Can you work these out from the model? Positions are in its coordinate system, mm. Face numbers are marked on the shaded views. A direction names the side the tool comes from. Coordinates: 2 decimals unless noted, no trailing zeros. Order: outer loops, then holes, each group sorted by start corner. A loop starts at its lowest first (then second) coordinate and runs counter-clockwise, first axis right, second up. Notation, with made-up numbers: M -6.75,28.5 L 45.25,28.5 A22 ccw 45.25,50.5 Z; hole C 8.25,9 d7. An arc over 180 degrees is marked long. Answer as a JSON object with one key per item and string values.
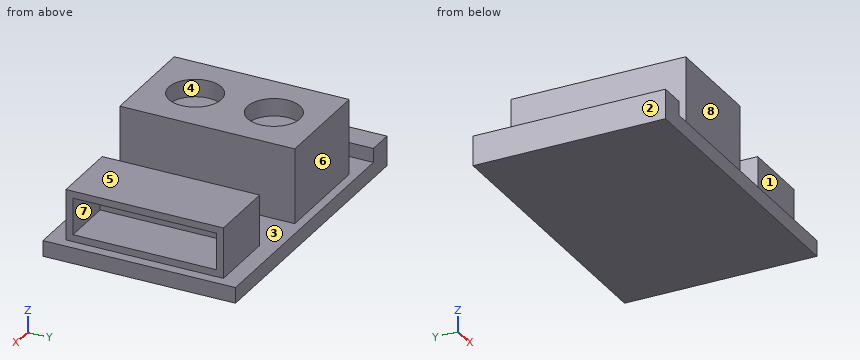
from build123d import *

# Parameters (mm, degrees)
ESBO_O1_W                = 16.7
ESBO_O1_H                = 11
RESSALTO_EXTRUS_O1_DEPTH = 5.2
ESBO_O2_W                = 16.7
ESBO_O2_H                = 11
ESBO_O2_W_2              = 6
ESBO_O2_H_2              = 10
ESBO_O2_W_3              = 4
ESBO_O2_H_3              = 9
CORTE_EXTRUS_O1_DEPTH    = 4.3
ESBO_O3_W                = 4
ESBO_O3_H                = 9
CORTE_EXTRUS_O2_DEPTH    = 1.4
ESBO_O4_R                = 1.5
CORTE_EXTRUS_O3_DEPTH    = 1
ESBO_O5_W                = 2.1
ESBO_O5_H                = 8.2
CORTE_EXTRUS_O4_DEPTH    = 3
ESBO_O6_W                = 1.5
ESBO_O6_H                = 11
RESSALTO_EXTRUS_O2_DEPTH = 0.8


with BuildPart() as part:
    # Esboço1 → Ressalto-extrusão1 (new body)
    with BuildSketch(Plane.XY):
        with Locations((3.068373494, 1.240361446)):
            Rectangle(ESBO_O1_W, ESBO_O1_H)
    extrude(amount=RESSALTO_EXTRUS_O1_DEPTH)

    # Esboço2 → Corte-extrusão1 (cut)
    with BuildSketch(Plane.XY.offset(5.2)):
        with Locations((3.068373494, 1.240361446)):
            Rectangle(ESBO_O2_W, ESBO_O2_H)
        with Locations((0.918373494, 1.240361446)):
            Rectangle(ESBO_O2_W_2, ESBO_O2_H_2, mode=Mode.SUBTRACT)
        with Locations((8.818373494, 1.240361446)):
            Rectangle(ESBO_O2_W_3, ESBO_O2_H_3, mode=Mode.SUBTRACT)
    extrude(amount=-CORTE_EXTRUS_O1_DEPTH, mode=Mode.SUBTRACT)

    # Esboço3 → Corte-extrusão2 (cut)
    with BuildSketch(Plane.XY.offset(5.2)):
        with Locations((8.818373494, 1.240361446)):
            Rectangle(ESBO_O3_W, ESBO_O3_H)
    extrude(amount=-CORTE_EXTRUS_O2_DEPTH, mode=Mode.SUBTRACT)

    # Esboço4 → Corte-extrusão3 (cut)
    with BuildSketch(Plane.XY.offset(5.2)):
        with Locations((0.918373494, 3.490361446)):
            Circle(ESBO_O4_R)
        with Locations((0.918373494, -1.009638554)):
            Circle(ESBO_O4_R)
    extrude(amount=-CORTE_EXTRUS_O3_DEPTH, mode=Mode.SUBTRACT)

    # Esboço5 → Corte-extrusão4 (cut)
    with BuildSketch(Plane(origin=(10.818373494, 0, 0), x_dir=(0, 0, -1), z_dir=(1, 0, 0))):
        with Locations((-2.35, 1.240361446)):
            Rectangle(ESBO_O5_W, ESBO_O5_H)
    extrude(amount=-CORTE_EXTRUS_O4_DEPTH, mode=Mode.SUBTRACT)

    # Esboço6 → Ressalto-extrusão2 (add)
    with BuildSketch(Plane.XY.offset(0.9)):
        with Locations((-4.531626506, 1.240361446)):
            Rectangle(ESBO_O6_W, ESBO_O6_H)
    extrude(amount=RESSALTO_EXTRUS_O2_DEPTH)


solid = part.part
Item 1: I want a section at B-B, the plane z = 2. Write out the boundary of the cut face in (x, y), plus the area to 3 significant figures.
Answers follow:
{"outline": "M -2.08,-3.76 L 3.92,-3.76 L 3.92,6.24 L -2.08,6.24 Z; M 6.82,-3.26 L 10.82,-3.26 L 10.82,-2.86 L 7.82,-2.86 L 7.82,5.34 L 10.82,5.34 L 10.82,5.74 L 6.82,5.74 Z", "area": "71.4 mm^2"}
Item 2: I want a section at A-A, the plane x = 8.75. Write out the boundary of the cut face in (y, z).
Answers follow:
{"outline": "M -4.26,0 L 6.74,0 L 6.74,0.9 L 5.74,0.9 L 5.74,3.8 L -3.26,3.8 L -3.26,0.9 L -4.26,0.9 Z; hole M -2.86,1.3 L 5.34,1.3 L 5.34,3.4 L -2.86,3.4 Z"}
Item 3: Please list where these lines run through material, in increasing order: line 1 (Z direction, x = 10.25, y = -2); line 2 (X direction, y = 0.75, z = 3.5); line 3 (X direction, y = -2.5, z = 2.45).
Answers follow:
{"line 1": "z = 0 to 1.3, 3.4 to 3.8", "line 2": "x = -2.08 to 3.92, 6.82 to 10.82", "line 3": "x = -2.08 to 3.92, 6.82 to 7.82"}
Item 4: If we mould it in two halves opening along X, with no side actions, what happens to the marked faces 1, 2 and 3? For each: pulls with the +X half, pulls with the -X half, needs draft (parallel to the pull), parting line crosses it, or undercut.
Answers follow:
{"face 1": "needs draft", "face 2": "pulls with the -X half", "face 3": "undercut"}
Item 5: Which directions (+Z, -Z, +X, -X, +Y, -Y) give clear straight access to the entire face, cutting with the end or side of a thin tool? Please do the marked faces 4, 5, 6, 7 and 8.
Answers follow:
{"face 4": "+Z", "face 5": "+Z, +X, +Y, -Y", "face 6": "+Z, +X, +Y", "face 7": "+X", "face 8": "+Z, +X, -Y"}
Item 6: I want a section at C-C, the plane y = 6. Write out the boundary of the cut face in (x, z), plus the area to 3 significant figures.
Answers follow:
{"outline": "M -5.28,0 L 11.42,0 L 11.42,0.9 L 3.92,0.9 L 3.92,5.2 L -2.08,5.2 L -2.08,0.9 L -3.78,0.9 L -3.78,1.7 L -5.28,1.7 Z", "area": "42.0 mm^2"}
Item 7: I want a section at D-D, the plane z = 4.55. Write out the boundary of the cut face in (x, y).
Answers follow:
{"outline": "M -2.08,-3.76 L 3.92,-3.76 L 3.92,6.24 L -2.08,6.24 Z; hole C 0.92,-1.01 d3; hole C 0.92,3.49 d3"}
Item 8: I'm going to push flat-ended pins straight in: pin 1 (2 mm diameter, centred on x = 1.5, z = 3, fed in from +Y); pin 2 (2.5 mm diameter, centred on y = -0.5, z = 2.5, fed in from -X); pin 3 (2 mm diameter, centred on y = 0.5, z = 4.5, fed in from -X); pin 4 (1.5 mm diameter, centred on x = 8.5, y = 0.5, fed in from +Z). Where does each tip first touch, or does it pass through?
Answers follow:
{"pin 1": "stops at y = 6.24", "pin 2": "stops at x = -5.28", "pin 3": "stops at x = -2.08", "pin 4": "stops at z = 3.8"}
